The model under review builds one solid part; all positions refer to its coordinate system, in mm. Round coordinates to 2 decimals unless told otherwise and drop trailing zeros. Write each loop counter-clockwise with the first axis right and the second up, starting at its lowest first coordinate (ties: lowest second). Pieces come first, ordered by that corner, then holes. Notation, with made-up numbers: (-19.5, -6.5) -> (18.5, -6.5) arc R19 ccw to (18.5, -1.5) -> close; hole circle Ø8 at (21, 16.25). An arc over 180 degrees is marked (long way). Return JSON: item names as keys, results as strings. Group by question number.
1. Take a section at B-B, the plane z = 1.95. Give the number of separate pieces and of enclosed holes in the cut face, then the cut area to 3 significant figures.
2. Take a section at A-A, the plane x = 81.5. Write out the cut boundary in (y, z), then the cut area to 3 significant figures.
3. For line 1 along X through (y, z) = (56, 2.2); line 2 along Y through (x, z) = (6, 1.05); line 3 along Y through (x, z) = (-26, 1.55), list the stretches that pass through material, from the lowest coordinate up. Write a range as from..to.
4. Clearance check with flat-ended pins moving along their axes: P1, Ø4, axis at x = 40, y = -60, coming from the -Z side; P2, Ø2, axis at x = -33, z = 1.5, coming from the -Y side; P3, Ø1.2, axis at y = 39.5, z = 2, coming from the +X side; P4, Ø2, axis at y = -57.5, z = 1.5, coming from the -X side. State where each tip first meets the part, or that it passes through.
from build123d import *

# Parameters (mm, degrees)
SKETCH_1_W          = 110
SKETCH_1_H          = 100
SKETCH_1_W_2        = 30
SKETCH_1_H_2        = 30
EXTRUDE_1_DEPTH     = 4
FILLET_1_R          = 50
SKETCH_2_R          = 13.5
SKETCH_2_R_2        = 1.5
CUT_EXTRUDE_1_DEPTH = 4
SKETCH_4_W          = 55
SKETCH_4_H          = 20
EXTRUDE_2_DEPTH     = 4
FILLET_2_R          = 5
SKETCH_5_R          = 1.5
CUT_EXTRUDE_2_DEPTH = 4


with BuildPart() as part:
    # 草图1 → 凸台-拉伸1 (new body)
    with BuildSketch(Plane.XY):
        Rectangle(SKETCH_1_W, SKETCH_1_H)
        Polygon((55, 70), (55, 50), (55, -50), (55, -70), (119, -70), (119, -15), (119, 15), (119, 70), align=None)
        with Locations((134, 0)):
            Rectangle(SKETCH_1_W_2, SKETCH_1_H_2)
    extrude(amount=EXTRUDE_1_DEPTH)

    # 圆角1
    fillet_1_edges = [part.edges().sort_by_distance(p)[0] for p in [
        (-55, -50, 2),
        (-55, 50, 2),
    ]]
    fillet(fillet_1_edges, radius=FILLET_1_R - 0.0001)  # a hair under: the kernel refuses the full size

    # 草图2 → 切除-拉伸1 (cut)
    with BuildSketch(Plane.XY.offset(4)):
        with BuildLine():
            ThreePointArc((7.5, 0), (-2.446129454, 12.236328912), (-16.456439237, 5))
            Line((-16.456439237, 5), (-7.5, 5))
            Line((-7.5, 5), (-7.5, -5))
            Line((-7.5, -5), (-16.456439237, -5))
            ThreePointArc((-16.456439237, -5), (-2.446129454, -12.236328912), (7.5, 0))
        make_face()
        with BuildLine():
            Line((-7.5, 5), (-16.456439237, 5))
            ThreePointArc((-16.456439237, 5), (-17.5, 0), (-16.456439237, -5))
            Line((-16.456439237, -5), (-7.5, -5))
            Line((-7.5, -5), (-7.5, 5))
        make_face()
        with BuildLine():
            Line((-16.456439237, 5), (-27.5, 5))
            Line((-27.5, 5), (-27.5, -5))
            Line((-27.5, -5), (-16.456439237, -5))
            ThreePointArc((-16.456439237, -5), (-17.5, 0), (-16.456439237, 5))
        make_face()
        with Locations((87, 36.5)):
            Circle(SKETCH_2_R)
        with Locations((99.374368671, 24.125631329)):
            Circle(SKETCH_2_R_2)
        with Locations((74.625631329, 24.125631329)):
            Circle(SKETCH_2_R_2)
        with Locations((74.625631329, 48.874368671)):
            Circle(SKETCH_2_R_2)
        with Locations((99.374368671, 48.874368671)):
            Circle(SKETCH_2_R_2)
        with Locations((87, -36.5)):
            Circle(SKETCH_2_R)
        with Locations((74.625631329, -24.125631329)):
            Circle(SKETCH_2_R_2)
        with Locations((99.374368671, -24.125631329)):
            Circle(SKETCH_2_R_2)
        with Locations((99.374368671, -48.874368671)):
            Circle(SKETCH_2_R_2)
        with BuildLine():
            ThreePointArc((-55, 0), (-54.937303656, 2.503138753), (-54.749371855, 5))
            Line((-54.749371855, 5), (-85.65404948, 5))
            Line((-85.65404948, 5), (-85.65404948, -5))
            Line((-85.65404948, -5), (-54.749371855, -5))
            ThreePointArc((-54.749371855, -5), (-54.937303656, -2.503138753), (-55, 0))
        make_face()
        with BuildLine():
            Line((-27.5, -5), (-27.5, 5))
            Line((-27.5, 5), (-54.749371855, 5))
            ThreePointArc((-54.749371855, 5), (-54.937303656, 2.503138753), (-55, 0))
            ThreePointArc((-55, 0), (-54.937303656, -2.503138753), (-54.749371855, -5))
            Line((-54.749371855, -5), (-27.5, -5))
        make_face()
        with Locations((74.625631329, -48.874368671)):
            Circle(SKETCH_2_R_2)
    extrude(amount=-CUT_EXTRUDE_1_DEPTH, mode=Mode.SUBTRACT)

    # 草图4 → 凸台-拉伸2 (add)
    with BuildSketch(Plane.XY.offset(4)):
        with Locations((27.5, 60)):
            Rectangle(SKETCH_4_W, SKETCH_4_H)
        with Locations((27.5, -60)):
            Rectangle(SKETCH_4_W, SKETCH_4_H)
    extrude(amount=-EXTRUDE_2_DEPTH)

    # 圆角2
    fillet_2_edges = [part.edges().sort_by_distance(p)[0] for p in [
        (0, -70, 2),
        (119, -70, 2),
        (119, -15, 2),
        (149, -15, 2),
        (149, 15, 2),
        (119, 15, 2),
        (119, 70, 2),
        (0, 50, 2),
        (-54.749381402, 5, 2),
        (-16.456439237, 5, 2),
        (-16.456439237, -5, 2),
        (-54.749381402, -5, 2),
        (0, -50, 2),
        (0, 70, 2),
    ]]
    fillet(fillet_2_edges, radius=FILLET_2_R)

    # 草图5 → 切除-拉伸2 (cut)
    with BuildSketch(Plane.XY.offset(4)):
        with Locations((114.5, 14)):
            Circle(SKETCH_5_R)
        with Locations((114.5, -14)):
            Circle(SKETCH_5_R)
        with Locations((69, 0)):
            Circle(SKETCH_5_R)
        with Locations((-36.819805153, 31.819805153)):
            Circle(SKETCH_5_R)
        with Locations((26.819805153, 31.819805153)):
            Circle(SKETCH_5_R)
        with Locations((26.819805153, -31.819805153)):
            Circle(SKETCH_5_R)
        with Locations((-36.819805153, -31.819805153)):
            Circle(SKETCH_5_R)
        with Locations((5, -60)):
            Circle(SKETCH_5_R)
        with Locations((20, -60)):
            Circle(SKETCH_5_R)
        with Locations((40, -60)):
            Circle(SKETCH_5_R)
        with Locations((5, 60)):
            Circle(SKETCH_5_R)
        with Locations((17, 60)):
            Circle(SKETCH_5_R)
        with Locations((44, 60)):
            Circle(SKETCH_5_R)
    extrude(amount=-CUT_EXTRUDE_2_DEPTH, mode=Mode.SUBTRACT)


solid = part.part
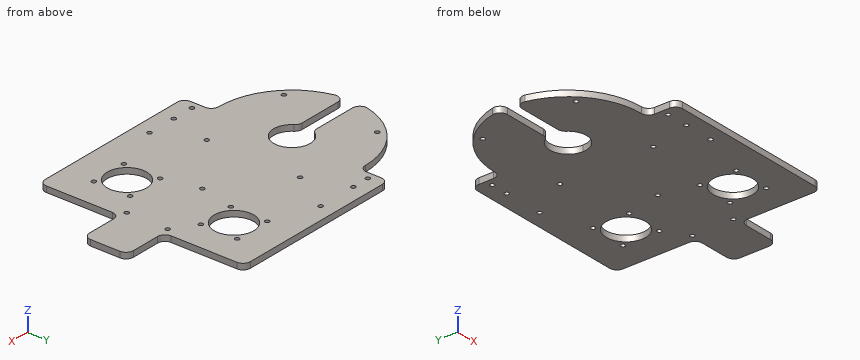
Output:
{
 "1": {"separate pieces": "1", "enclosed holes": "23", "area": "19,800 mm^2"},
 "2": {"outline": "(-70, 0) -> (-48.83, 0) -> (-48.83, 4) -> (-70, 4) -> close; (-24.17, 0) -> (24.17, 0) -> (24.17, 4) -> (-24.17, 4) -> close; (48.83, 0) -> (70, 0) -> (70, 4) -> (48.83, 4) -> close", "area": "363 mm^2"},
 "3": {"line 1": "x = 0..119", "line 2": "y = -70..-61.12, -58.88..-5.94, 5.94..58.88, 61.12..70", "line 3": "y = -45.38..-5, 5..45.38"},
 "4": {"P1": "stops at z = 0", "P2": "stops at y = -42.08", "P3": "stops at x = 119", "P4": "stops at x = 0"}
}
